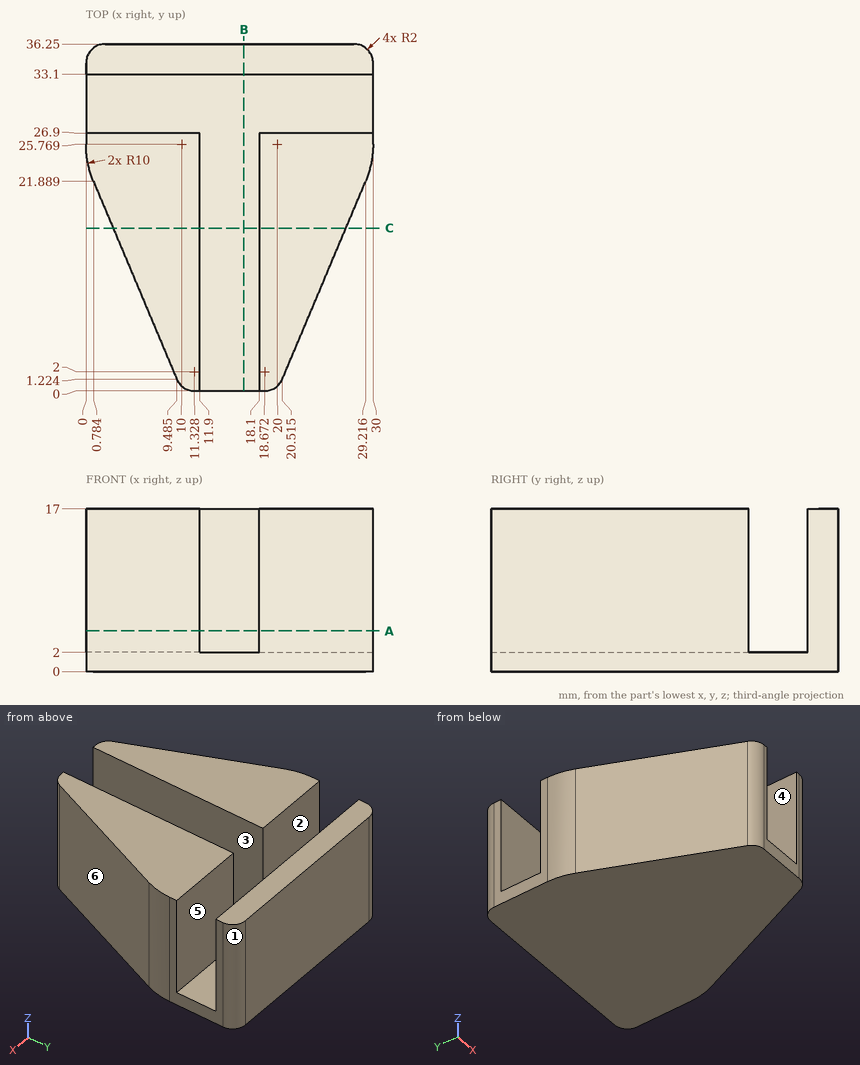
Can you work these out from the drawing? Everything is in mm from the part's minimum corner. A direction names the side the tool comes from. Round coordinates to 2 decimals unless told otherwise and drop trailing zeros. Order: outer loops, then holes, each group sorted by start corner. A loop starts at its lowest first (then second) coordinate and runs counter-clockwise, first axis right, second up. Notation, with made-up numbers: (84.25, 35) -> (135.25, 35) arc R21 cw to (135.25, 53) -> close; hole circle Ø10 at (60.5, 19). An arc over 180 degrees is marked (long way). Return JSON: item names as keys, results as strings. Group by question number.
1. Which directions (+Z, -Z, +X, -X, +Y, -Y) give clear straight access to the entire face, cutting with the end or side of a thin tool? Please do the marked faces 1, 2 and 3.
2. We'd pull the mould along Y, two halves only. Please class the marked faces 4, 5 and 6: released by +Y, released by -Y, zero draft, split by the parting line, or undercut.
3. I need wall thicknesses on line 1 (Z direction, x = 18.75, y = 27); line 2 (X direction, y = 13, z = 7.5) (1 decimal); line 3 (Y direction, x = 2, z = 10). Which ranges of each line are inside material? Lowest first, please. Write a range as [from, to].
4. If we section it at B-B, the plane x = 16.5: Write out the boundary of the cut face in (y, z).
5. Will these pins go through, and if not, where does the flat tip stop? pin 1 (2 mm diameter, centred on y = 18.5, z = 8.5, fed in from -X); pin 2 (1.5 mm diameter, centred on x = 22, z = 10.5, fed in from -Y).
6. If we section it at A-A, the plane z = 4.25: Count the separate pieces of the cut face and the enclosed holes in it.
7. If we section it at C-C, the plane y = 17: Write out the boundary of the cut face in (x, z), then the cut area to 3 significant figures.
Output values:
{
 "1": {"face 1": "+Z, -Z, +X, +Y", "face 2": "+Z, +X, -X", "face 3": "+Z, -Y"},
 "2": {"face 4": "zero draft", "face 5": "undercut", "face 6": "released by -Y"},
 "3": {"line 1": "[0, 2]", "line 2": "[4.5, 11.9], [18.1, 25.5]", "line 3": "[19, 26.9], [33.1, 36.25]"},
 "4": {"outline": "(0, 0) -> (36.25, 0) -> (36.25, 17) -> (33.1, 17) -> (33.1, 2) -> (0, 2) -> close"},
 "5": {"pin 1": "x = 1.79", "pin 2": "y = 2.97"},
 "6": {"separate pieces": "3", "enclosed holes": "0"},
 "7": {"outline": "(2.84, 0) -> (27.16, 0) -> (27.16, 17) -> (18.1, 17) -> (18.1, 2) -> (11.9, 2) -> (11.9, 17) -> (2.84, 17) -> close", "area": "320 mm²"}
}
